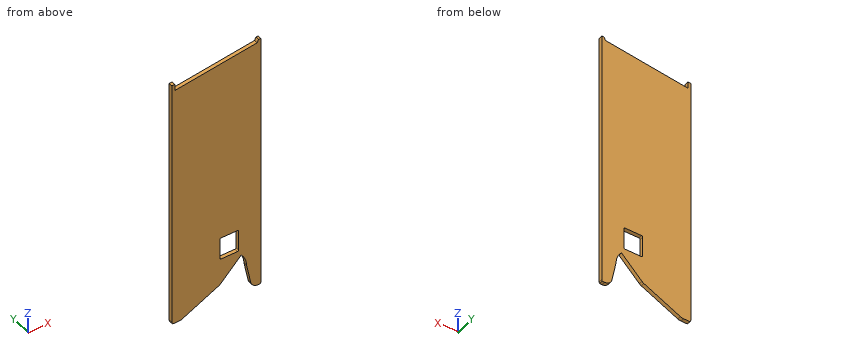
```python
from build123d import *

# Parameters (mm, degrees)
SKETCH1_W           = 609.6
SKETCH1_H           = 1828.8
BOSS_EXTRUDE1_DEPTH = 25.4
FILLET1_R           = 25.4
CUT_EXTRUDE2_DEPTH  = 965.196847122
CUT_EXTRUDE3_DEPTH  = 965.196847122
CUT_EXTRUDE4_DEPTH  = 956.204611857


with BuildPart() as part:
    # Sketch1 → Boss-Extrude1 (new body)
    with BuildSketch(Plane(origin=(0, 0, 0), x_dir=(1, 0, 0), z_dir=(0, 1, 0))):
        Rectangle(SKETCH1_W, SKETCH1_H)
    extrude(amount=BOSS_EXTRUDE1_DEPTH)

    # Fillet1
    fillet1_edges = [part.edges().sort_by_distance(p)[0] for p in [
        (-304.8, 12.7, -914.4),
        (304.8, 12.7, -914.4),
        (304.8, 12.7, 914.4),
        (-304.8, 12.7, 914.4),
    ]]
    fillet(fillet1_edges, radius=FILLET1_R)

    # Sketch3 → Cut-Extrude2 (cut, through all)
    with BuildSketch(Plane(origin=(0, 25.4, 0), x_dir=(1, 0, 0), z_dir=(0, 1, 0))):
        with BuildLine():
            Line((16.251587569, 779.193092163), (-233.147514188, 899.843092163))
            ThreePointArc((-233.147514188, 899.843092163), (-243.921993823, 903.629350189), (-255.27, 904.913062406))
            Line((-255.27, 904.913062406), (-323.85, 904.913062406))
            Line((-323.85, 904.913062406), (-323.85, 931.593092163))
            Line((-323.85, 931.593092163), (311.15, 931.593092163))
            Line((311.15, 931.593092163), (311.15, 899.843092163))
            Line((311.15, 899.843092163), (285.75, 899.843092163))
            ThreePointArc((285.75, 899.843092163), (253.698373918, 888.455441312), (236.016540238, 859.397945134))
            Line((236.016540238, 859.397945134), (207.824095772, 723.992082179))
            ThreePointArc((207.824095772, 723.992082179), (207.109723344, 719.608512763), (206.78096626, 715.179299789))
            ThreePointArc((206.78096626, 715.179299789), (196.558100486, 668.783623502), (170.129901322, 629.30431181))
            Line((170.129901322, 629.30431181), (30.050126241, 769.384086891))
            ThreePointArc((30.050126241, 769.384086891), (23.562355365, 774.867453261), (16.251587569, 779.193092163))
        make_face()
    extrude(amount=-CUT_EXTRUDE2_DEPTH, mode=Mode.SUBTRACT)

    # Sketch4 → Cut-Extrude3 (cut, through all)
    with BuildSketch(Plane(origin=(0, 25.4, 0), x_dir=(1, 0, 0), z_dir=(0, 1, 0))):
        Polygon((-327.069996122, -833.12), (-283.889996122, -833.12), (-283.889996122, -788.67), (279.4, -864.87), (289.56, -885.19), (330.2, -885.19), (330.2, -946.15), (-327.069996122, -946.15), align=None)
    extrude(amount=-CUT_EXTRUDE3_DEPTH, mode=Mode.SUBTRACT)

    # Sketch5 → Cut-Extrude4 (cut, through all)
    with BuildSketch(Plane.XZ):
        with BuildLine():
            Line((152.843358649, -583.374519212), (152.843358649, -445.325480788))
            add(Edge.make_bspline(
                [(152.843358649, -445.325480788), (152.843358649, -437.706641351), (145.224519212, -437.706641351)],
                knots=[2.356346783, 2.356346783, 2.356346783, 3.926838524, 3.926838524, 3.926838524], degree=2, weights=[1, 0.707214461, 1]))
            Line((145.224519212, -437.706641351), (32.575480788, -437.706641351))
            add(Edge.make_bspline(
                [(32.575480788, -437.706641351), (24.956641351, -437.706641351), (24.956641351, -445.325480788)],
                knots=[2.356346783, 2.356346783, 2.356346783, 3.926838524, 3.926838524, 3.926838524], degree=2, weights=[1, 0.707214461, 1]))
            Line((24.956641351, -445.325480788), (24.956641351, -583.374519212))
            add(Edge.make_bspline(
                [(24.956641351, -583.374519212), (24.956641351, -590.993358649), (32.575480788, -590.993358649)],
                knots=[2.356346783, 2.356346783, 2.356346783, 3.926838524, 3.926838524, 3.926838524], degree=2, weights=[1, 0.707214461, 1]))
            Line((32.575480788, -590.993358649), (145.224519212, -590.993358649))
            add(Edge.make_bspline(
                [(145.224519212, -590.993358649), (152.843358649, -590.993358649), (152.843358649, -583.374519212)],
                knots=[2.356346783, 2.356346783, 2.356346783, 3.926838524, 3.926838524, 3.926838524], degree=2, weights=[1, 0.707214461, 1]))
        make_face()
    extrude(amount=-CUT_EXTRUDE4_DEPTH, mode=Mode.SUBTRACT)


solid = part.part
```
Source: CAD feature listing. Evaluate the final solid. Frame: model axes, mm. Coordinates: 2 decimals unless noted, no trailing zeros. Write each loop counter-clockwise with the first axis right and the second up, starting at its lowest first coordinate (ties: lowest second). Pieces come first, ordered by that corner, then holes. Notation, with made-up numbers: (0, -1.75) -> (52, -1.75) arc R22 ccw to (52, 27.25) -> close; hole circle Ø9 at (59, -16). An arc over 180 degrees is marked (long way). Return JSON: item names as keys, results as strings. Group by question number.
1) Contact query for flat-ended pins moving along their axis: P1, Ø3, axis at x = -241, y = 3.5, coming from the -Z side; P2, Ø8.5, axis at x = 294, y = 14.5, coming from the -Z side; P3, Ø10.5, axis at x = -290.5, y = 7.5, coming from the +Z side. Output: stop coordinate, or through.
2) Ray query, line 1 along X through (y, z) = (16, -516); line 2 along X through (y, z) = (11, -586); line 3 along Z through (x, y) = (120, 1.5). Return the intervals inside material, ascending.
3) Section query A-A, the plane z = -687.5. Return loops of the section in (x, y).
4) Section query B-B, the plane x = 120. Return loops of the section in (y, z).
5) Section query C-C, the plane x = -170.5. Return loops of the section in (y, z).
From the geometry:
{
 "1": {"P1": "z = -903.28", "P2": "z = -899.84", "P3": "z = 833.12"},
 "2": {"line 1": "-304.8 to 24.96, 152.84 to 304.8", "line 2": "-304.8 to 25.42, 152.38 to 304.8", "line 3": "-679.43 to -590.99, -437.71 to 843.31"},
 "3": {"outline": "(-304.8, 0) -> (111.93, 0) -> (111.93, 25.4) -> (-304.8, 25.4) -> close; (202.89, 0) -> (304.8, 0) -> (304.8, 25.4) -> (202.89, 25.4) -> close"},
 "4": {"outline": "(0, -679.43) -> (25.4, -679.43) -> (25.4, -590.99) -> (0, -590.99) -> close; (0, -437.71) -> (25.4, -437.71) -> (25.4, 843.31) -> (0, 843.31) -> close"},
 "5": {"outline": "(0, -869.54) -> (25.4, -869.54) -> (25.4, 804.01) -> (0, 804.01) -> close"}
}
